```python
from build123d import *

# Parameters (mm, degrees)
F0_W     = 279.4
F0_H     = 482.6
F1_DEPTH = 25.4
F3_DEPTH = 381
F4_T     = -2.54


with BuildPart() as f1:
    # F0 (on Front) → F1 (new body)
    with BuildSketch(Plane.XZ):
        with Locations((-116.0904299468, 41.1734286772)):
            Rectangle(F0_W, F0_H)
    extrude(amount=F1_DEPTH)

    # F3 (add): a face of the model
    f3_faces = [f1.faces().sort_by_distance(p)[0] for p in [
        (-116.0904299468, -25.4, 41.1734286772),
    ]]
    extrude(f3_faces, amount=F3_DEPTH)

    # F4
    f4_openings = [f1.faces().sort_by_distance(p)[0] for p in [
        (-116.09043, -406.4, 41.173429),
    ]]
    offset(amount=F4_T, openings=f4_openings)


solid = f1.part
```
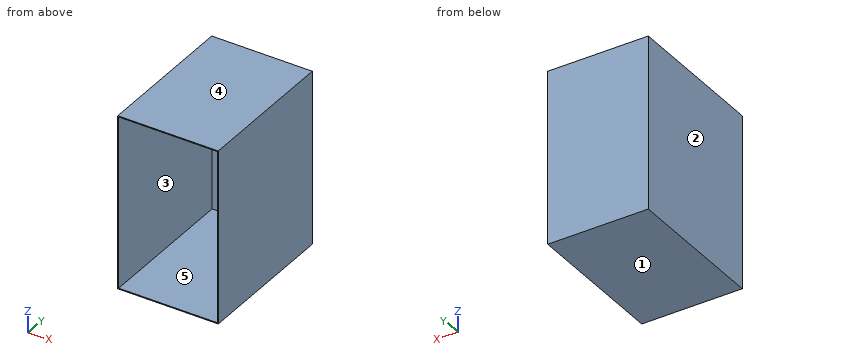
Build history of the part. All positions in model axes, mm. Face numbers are marked on the shaded views. A direction names the side the tool comes from. Give positions to 0.01 mm unless a question says otherwise; leave off trailing zeros. Loops run counter-clockwise (first coordinate to the right, second up) from the corner with the lowest first, then second, coordinate; pieces in that order, holes last. Notation, with made-up numbers: (-27, 68) -> (-4, 68) arc R25 cw to (-4, 81) -> close; hole circle Ø2 at (27, 75). An arc over 180 degrees is marked (long way). One line per question, with ' | ' between items. Start each with the question number.
1) Probe L1, parallel to X at y = -357, z = -157; L2, parallel to Z at x = -65, y = -87; L3, parallel to Y at x = -199.5, z = 120.5. List the from-to ranges inside material, lowest first.
2) Two-plate mould, pull along X, no slides. Class the marked faces 1, 2 and 3: released by +X, released by -X, zero draft, split by the parting line, or undercut.
3) 3-axis set-ups, long thin cutter, end or side, ignore diameter. For the marked faces 4 and 5: which of +Z, -Z, +X, -X, +Y, -Y reach the whole face in a straight line?
4) Cut at C-C (z = -112). Give the cut face in (x, y).
5) Cut at A-A (y = -63). Give the cut face in (x, z), plus the area to 3 significant figures.
6) Cut at B-B (x = -227). Give the cut face in (y, z).
7) Pin check, flat tips, straight feed: pin 1 (6 mm diameter, centred on x = -84, z = 83.5, fed in from -Y); pin 2 (1 mm diameter, centred on x = -120, z = 216, fed in from +Y). Stop position of each tip, or through.
Return value:
1) L1: -255.79 to -253.25, 21.07 to 23.61 | L2: -200.13 to -197.59, 279.93 to 282.47 | L3: -2.54 to 0
2) face 1: zero draft | face 2: released by -X | face 3: undercut
3) face 4: +Z, +X, -X, +Y, -Y | face 5: -Y
4) outline: (-255.79, -406.4) -> (-253.25, -406.4) -> (-253.25, -2.54) -> (21.07, -2.54) -> (21.07, -406.4) -> (23.61, -406.4) -> (23.61, 0) -> (-255.79, 0) -> close
5) outline: (-255.79, -200.13) -> (23.61, -200.13) -> (23.61, 282.47) -> (-255.79, 282.47) -> close; hole (-253.25, -197.59) -> (21.07, -197.59) -> (21.07, 279.93) -> (-253.25, 279.93) -> close | area: 3,850 mm^2
6) outline: (-406.4, -200.13) -> (0, -200.13) -> (0, 282.47) -> (-406.4, 282.47) -> (-406.4, 279.93) -> (-2.54, 279.93) -> (-2.54, -197.59) -> (-406.4, -197.59) -> close
7) pin 1: y = -2.54 | pin 2: y = 0
